from build123d import *

# Parameters (mm, degrees)
SKETCH1_R                 = 50
SKETCH1_R_2               = 30
BOSS_EXTRUDE1_DEPTH       = 20
CHAMFER1_SIZE             = 5
M6X1_0_TAPPED_HOLE1_D     = 5
M6X1_0_TAPPED_HOLE1_DEPTH = 50
M6X1_0_TAPPED_HOLE1_TIP   = 1.502151548
SKETCH4_R                 = 5
CUT_EXTRUDE1_DEPTH        = 6


with BuildPart() as part:
    # Sketch1 → Boss-Extrude1 (new body)
    with BuildSketch(Plane(origin=(0, 0, 0), x_dir=(1, 0, 0), z_dir=(0, 1, 0))):
        with Locations(Location((0, 0, 0), (0, 0, 270))):
            Circle(SKETCH1_R)
        with Locations(Location((0, 0, 0), (0, 0, 270))):
            Circle(SKETCH1_R_2, mode=Mode.SUBTRACT)
    extrude(amount=BOSS_EXTRUDE1_DEPTH)

    # Chamfer1
    chamfer1_edges = [part.edges().sort_by_distance(p)[0] for p in [
        (0, 20, -50),
    ]]
    chamfer(chamfer1_edges, length=CHAMFER1_SIZE)

    # M6x1.0 Tapped Hole1
    with Locations(Plane(origin=(-37, 20, 0), x_dir=(0, 0, 1), z_dir=(0, 1, 0))):
        with Locations((0, 0), (0, 74)):
            Hole(M6X1_0_TAPPED_HOLE1_D / 2, depth=M6X1_0_TAPPED_HOLE1_DEPTH)
            with Locations((0, 0, -(M6X1_0_TAPPED_HOLE1_DEPTH + M6X1_0_TAPPED_HOLE1_TIP / 2))):  # 118° drill point
                Cone(0, M6X1_0_TAPPED_HOLE1_D / 2, M6X1_0_TAPPED_HOLE1_TIP, mode=Mode.SUBTRACT)

    # Sketch4 → Cut-Extrude1 (cut)
    with BuildSketch(Plane(origin=(0, 20, 0), x_dir=(1, 0, 0), z_dir=(0, 1, 0))):
        with Locations(Location((-37, 0, 0), (0, 0, 270))):
            Circle(SKETCH4_R)
        with Locations(Location((37, 0, 0), (0, 0, 270))):
            Circle(SKETCH4_R)
    extrude(amount=-CUT_EXTRUDE1_DEPTH, mode=Mode.SUBTRACT)


solid = part.part
The model under review builds one solid part; all positions refer to its coordinate system, in mm. A direction names the side the tool comes from. Round coordinates to 2 decimals unless told otherwise and drop trailing zeros. Loops run counter-clockwise (first coordinate to the right, second up) from the corner with the lowest first, then second, coordinate; pieces in that order, holes last. Notation, with made-up numbers: (-13.75, 17) -> (26.25, 17) arc R28 ccw to (26.25, 36) -> close; hole circle Ø10 at (26, 25.25). An arc over 180 degrees is marked (long way). One line per question, with ' | ' between items. Start each with the question number.
Item 1: For pin 1 (5 mm diameter, centred on y = 17.5, z = -27, fed in from +X); pin 2 (2 mm diameter, centred on y = 16.5, z = -15.5, fed in from +X); pin 3 (1.5 mm diameter, centred on x = 19.5, y = 9.5, fed in from +Z), all flat-tipped, find the tip position at first contact; note any pin that passes through.
Item 2: Machinability: for faces 1 (the face through (-39, 14, 2)), 2 (the face through (-39.44, 6.9, 0.54)), which of the approach directions +Z, -Z, +X, -X, +Y, -Y give a long, thin tool a straight path to every point of the face, cutting with its end or side? Answer none if there is none.
Item 3: Draft analysis for pull direction X (two halves, no side actions). For faces 3 (the face through (-9, 20, 29)), 4 (the face through (-32.043, 17.042, -0.651)), 5 (the face through (15.02, 7.4, 47.69)), 6 (the face through (35, 14, 2)), state which applies: +X half, -X half, draft (parallel to the pull), parting line (faces both ways), or undercut.
Item 4: Add section A-A, the plane z = 0. Write out the cut boundary in (x, y).
Item 5: Add section C-C, the plane y = 17. Write out the cut boundary in (x, z).
Item 6: Add section D-D, the plane y = 4.5. Write out the cut boundary in (x, z).
Item 7: Wall thickness on line 1 along X through (y, z) = (7.75, 0); line 2 along X through (y, z) = (16, 0); line 3 along X through (y, z) = (14, -14): over which ranges is each line inside the solid? List them lowest first. Write a range as [from, to].
Item 8: Add section B-B, the plane x = 0. Write out the cut boundary in (y, z).
Return value:
1) pin 1: stops at x = 42.47 | pin 2: stops at x = 47.06 | pin 3: stops at z = 46.35
2) face 1: +Y | face 2: +Y, -Y
3) face 3: draft | face 4: undercut | face 5: parting line | face 6: undercut
4) outline: (-50, 0) -> (-39.5, 0) -> (-39.5, 14) -> (-42, 14) -> (-42, 20) -> (-45, 20) -> (-50, 15) -> close; (-34.5, 0) -> (-30, 0) -> (-30, 20) -> (-32, 20) -> (-32, 14) -> (-34.5, 14) -> close; (30, 0) -> (34.5, 0) -> (34.5, 14) -> (32, 14) -> (32, 20) -> (30, 20) -> close; (39.5, 0) -> (50, 0) -> (50, 15) -> (45, 20) -> (42, 20) -> (42, 14) -> (39.5, 14) -> close
5) outline: circle Ø96 at (0, 0); hole circle Ø10 at (-37, 0); hole circle Ø60 at (0, 0); hole circle Ø10 at (37, 0)
6) outline: circle Ø100 at (0, 0); hole circle Ø5 at (-37, 0); hole circle Ø60 at (0, 0); hole circle Ø5 at (37, 0)
7) line 1: x = [-50, -39.5], [-34.5, -30], [30, 34.5], [39.5, 50] | line 2: x = [-49, -42], [-32, -30], [30, 32], [42, 49] | line 3: x = [-48, -26.53], [26.53, 48]
8) outline: (0, -50) -> (15, -50) -> (20, -45) -> (20, -30) -> (0, -30) -> close; (0, 30) -> (20, 30) -> (20, 45) -> (15, 50) -> (0, 50) -> close
